Part model, mm, in its own coordinate system. Face numbers are marked on the shaded views. A direction names the side the tool comes from. Give positions to 0.01 mm unless a question says otherwise; leave off trailing zeros. Order: outer loops, then holes, each group sorted by start corner. A loop starts at its lowest first (then second) coordinate and runs counter-clockwise, first axis right, second up. Notation, with made-up numbers: M 83.25,27 L 132.25,27 A19 ccw 132.25,59 Z; hole C -0.75,-3 d6. An arc over 180 degrees is marked long. Answer as a JSON object with one key per item and string values.
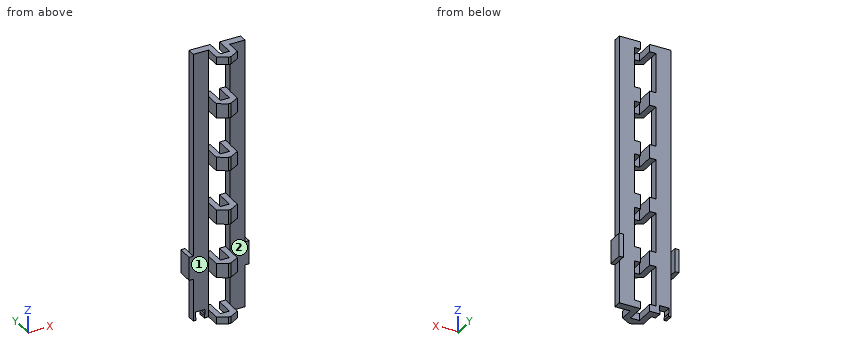
Autodesk Inventor part; units mm, degrees
ref_plane "p1_XY" through (0, 0, 0) normal (0, 1, 0) x (1, 0, 0)
ref_plane "p1_YZ" through (0, 0, 0) normal (1, 0, 0) x (0, 0, -1)
ref_plane "p1_ZX" through (0, 0, 0) normal (0, 0, -1) x (0, 1, 0)
sketch "Sketch_1" plane through (0, 0, 0) normal (0, 0, 1) x (1, 0, 0)
  line L0 (-17, 17.82) -> (-17, 12.62)
  line L1 (-17, 12.62) -> (-6.9, 12.62)
  line L2 (-6.9, 12.62) -> (-6.9, 3.4641)
  line L3 (-6.9, 3.4641) -> (-0.9, 0)
  line L4 (-0.9, 0) -> (0.9, 0)
  line L5 (0.9, 0) -> (6.9, 3.4641)
  line L6 (6.9, 3.4641) -> (6.9, 12.62)
  line L7 (6.9, 12.62) -> (17, 12.62)
  line L8 (17, 12.62) -> (17, 17.82)
  line L9 (17, 17.82) -> (3, 17.82)
  line L10 (3, 17.82) -> (3, 5.67)
  line L11 (3, 5.67) -> (-3, 5.67)
  line L12 (-3, 5.67) -> (-3, 17.82)
  line L13 (-3, 17.82) -> (-17, 17.82)
extrude "Extrusion1" add sketch "Sketch_1" along normal blind 178
sketch "Sketch_9" plane through (0, 0, 0) normal (0, 1, 0) x (-1, 0, 0)
  line L0 (7.12, 4.62) -> (7.12, 30.82)
  line L1 (7.12, 30.82) -> (-7.12, 30.82)
  line L2 (-7.12, 30.82) -> (-7.12, 4.62)
  line L3 (-7.12, 4.62) -> (7.12, 4.62)
extrude "Extrusion2" cut sketch "Sketch_9" along normal blind 25
sketch "Sketch_2" plane through (0, 0, 0) normal (0, 1, 0) x (-1, 0, 0)
  line L0 (7.12, 40.33) -> (7.12, 66.53)
  line L1 (7.12, 66.53) -> (-7.12, 66.53)
  line L2 (-7.12, 66.53) -> (-7.12, 40.33)
  line L3 (-7.12, 40.33) -> (7.12, 40.33)
extrude "Extrusion3" cut sketch "Sketch_2" along normal blind 25
sketch "Sketch_3" plane through (0, 0, 0) normal (0, 1, 0) x (-1, 0, 0)
  line L0 (7.12, 76.04) -> (7.12, 102.24)
  line L1 (7.12, 102.24) -> (-7.12, 102.24)
  line L2 (-7.12, 102.24) -> (-7.12, 76.04)
  line L3 (-7.12, 76.04) -> (7.12, 76.04)
extrude "Extrusion4" cut sketch "Sketch_3" along normal blind 25
sketch "Sketch_4" plane through (0, 0, 0) normal (0, 1, 0) x (-1, 0, 0)
  line L0 (7.12, 111.21) -> (7.12, 137.41)
  line L1 (7.12, 137.41) -> (-7.12, 137.41)
  line L2 (-7.12, 137.41) -> (-7.12, 111.21)
  line L3 (-7.12, 111.21) -> (7.12, 111.21)
extrude "Extrusion5" cut sketch "Sketch_4" along normal blind 25
sketch "Sketch_5" plane through (0, 0, 0) normal (0, 1, 0) x (-1, 0, 0)
  line L0 (7.12, 146.92) -> (7.12, 173.12)
  line L1 (7.12, 173.12) -> (-7.12, 173.12)
  line L2 (-7.12, 173.12) -> (-7.12, 146.92)
  line L3 (-7.12, 146.92) -> (7.12, 146.92)
extrude "Extrusion6" cut sketch "Sketch_5" along normal blind 25
sketch "Sketch_12" plane through (17, 17.82, 0) normal (0, 1, 0) x (-1, 0, 0)
  line L0 (26.3, 5.6) -> (26.3, 2.5)
  line L1 (26.3, 2.5) -> (26.8, 1.6)
  line L2 (26.8, 1.6) -> (26.8, 0)
  line L3 (26.8, 0) -> (32.2, 0)
  line L4 (32.2, 0) -> (32.2, 1.6)
  line L5 (32.2, 1.6) -> (32.7, 2.5)
  line L6 (32.7, 2.5) -> (32.7, 5.6)
  line L7 (32.7, 5.6) -> (26.3, 5.6)
extrude "Extrusion8" cut sketch "Sketch_12" against normal blind 6
sketch "Sketch_16" plane through (-17, 12.62, 0) normal (-1, 0, 0) x (0, 0, 1)
  line L0 (27.9, 10) -> (27.9, 0)
  line L1 (27.9, 0) -> (43.3, 0)
  line L2 (43.3, 0) -> (43.3, 10)
  line L3 (43.3, 10) -> (27.9, 10)
extrude "Extrusion9" add sketch "Sketch_16" along normal blind 2.75
sketch "Sketch_14" plane through (17, 17.82, 0) normal (1, 0, 0) x (0, 0, 1)
  line L0 (27.9, -4.8) -> (43.3, -4.8)
  line L1 (43.3, -4.8) -> (43.3, 5.2)
  line L2 (43.3, 5.2) -> (27.9, 5.2)
  line L3 (27.9, 5.2) -> (27.9, -4.8)
extrude "Extrusion10" add sketch "Sketch_14" along normal blind 2.75
ref_plane "p1_XY" through (0, 0, 0) normal (0, 1, 0) x (1, 0, 0)
ref_plane "p1_YZ" through (0, 0, 0) normal (1, 0, 0) x (0, 0, -1)
ref_plane "p1_ZX" through (0, 0, 0) normal (0, 0, -1) x (0, 1, 0)
properties part number "PRO10315 Rolle fuer Rollenleiste 178"
1. Cut at A-A on y = 20.5. Give the cut face in (x, z), plus the area to 3 significant figures.
Worked answers:
{"outline": "M -19.75,27.9 L -17,27.9 L -17,43.3 L -19.75,43.3 Z; M 17,27.9 L 19.75,27.9 L 19.75,43.3 L 17,43.3 Z", "area": "84.7 mm^2"}
2. Cut at B-B on z = 160.5. Give the cut face in (x, y).
Worked answers:
{"outline": "M -17,12.62 L -7.12,12.62 L -7.12,17.82 L -17,17.82 Z; M 7.12,12.62 L 17,12.62 L 17,17.82 L 7.12,17.82 Z"}
3. Pin check, flat tips, straight feed: P1, Ø5.5, axis at y = 16, z = 15, coming from the -X side; P2, Ø1.3, axis at y = 14, z = 1, coming from the +X side; P3, Ø1.5, axis at x = -11, y = 14, coming from the -Z side. Stop position of each tip, or through.
Worked answers:
{"P1": "stops at x = -17", "P2": "stops at x = 17", "P3": "stops at z = 5.6"}
4. Probe line 1 along Z through (x, y) = (4, 9.5); line 2 along X through (y, z) = (11.5, 32); line 3 along X through (y, z) = (13.75, 19). List the from-to ranges inside material, lowest first.
Worked answers:
{"line 1": "z = 0 to 4.62, 30.82 to 40.33, 66.53 to 76.04, 102.24 to 111.21, 137.41 to 146.92, 173.12 to 178", "line 2": "x = -6.9 to -3, 3 to 6.9", "line 3": "x = -17 to -7.12, 7.12 to 17"}
5. Which spindle directions (+Z, -Z, +X, -X, +Y, -Y) get a long thin tool onto all of the face, cutting with end or side? Do the marked faces 1 and 2. Say none if no direction does.
Worked answers:
{"face 1": "+Z, -Z, -X, -Y", "face 2": "+Z, -Z, +X, -Y"}
6. Cut at C-C on x = 4.5. Give the cut face in (y, z), plus the area to 3 significant figures.
Worked answers:
{"outline": "M 2.08,0 L 17.82,0 L 17.82,4.62 L 2.08,4.62 Z; M 2.08,30.82 L 17.82,30.82 L 17.82,40.33 L 2.08,40.33 Z; M 2.08,66.53 L 17.82,66.53 L 17.82,76.04 L 2.08,76.04 Z; M 2.08,102.24 L 17.82,102.24 L 17.82,111.21 L 2.08,111.21 Z; M 2.08,137.41 L 17.82,137.41 L 17.82,146.92 L 2.08,146.92 Z; M 2.08,173.12 L 17.82,173.12 L 17.82,178 L 2.08,178 Z", "area": "740 mm^2"}
7. Cut at D-D on z = 68. Give the cut face in (x, y), plus the area to 3 significant figures.
Worked answers:
{"outline": "M -17,12.62 L -6.9,12.62 L -6.9,3.46 L -0.9,0 L 0.9,0 L 6.9,3.46 L 6.9,12.62 L 17,12.62 L 17,17.82 L 3,17.82 L 3,5.67 L -3,5.67 L -3,17.82 L -17,17.82 Z", "area": "257 mm^2"}
